Source: CAD feature listing. Evaluate the final solid. Frame: model axes, mm. A direction names the side the tool comes from. Give positions to 0.01 mm unless a question says otherwise; leave off trailing zeros. Loops run counter-clockwise (first coordinate to the right, second up) from the corner with the lowest first, then second, coordinate; pieces in that order, holes last. Notation, with made-up numbers: M 1.5,40.5 L 42.5,40.5 A3 ccw 42.5,45.5 Z; hole C 78.25,43 d10. An arc over 180 degrees is marked long. Put each result on its own line as item: value.
from build123d import *

# Parameters (mm, degrees)
F0_W     = 82
F0_H     = 60.5
F1_DEPTH = 2
F2_R     = 2.375
F3_DEPTH = 2
F4_DEPTH = 4
F5_DEPTH = 2
F6_W     = 2
F6_H     = 10.75
F7_DEPTH = 10.501
F8_W     = 0.5
F8_H     = 10
F9_DEPTH = 5


with BuildPart() as f1:
    # F0 (on Top) → F1 (new body)
    with BuildSketch(Plane.XY):
        Rectangle(F0_W, F0_H)
    extrude(amount=F1_DEPTH)

    # F2 (on face) → F3 (join)
    with BuildSketch(Plane.YZ.offset(41)):
        Polygon((19.5, 2), (-19.5, 2), (-30.25, 2), (-30.25, 0), (30.25, 0), (30.25, 2), align=None)
        with BuildLine():
            Line((19.5, 7.125), (19.5, 2))
            Line((19.5, 2), (30.25, 2))
            Line((30.25, 2), (30.25, 7.125))
            ThreePointArc((30.25, 7.125), (24.875, 12.5), (19.5, 7.125))
        make_face()
        with Locations((24.875, 7.125)):
            Circle(F2_R, mode=Mode.SUBTRACT)
    extrude(amount=F3_DEPTH)

    # F2 (on face) → F4 (join)
    with BuildSketch(Plane.YZ.offset(41)):
        with BuildLine():
            Line((-30.25, 2), (-19.5, 2))
            Line((-19.5, 2), (-19.5, 7.125))
            ThreePointArc((-19.5, 7.125), (-24.875, 12.5), (-30.25, 7.125))
            Line((-30.25, 7.125), (-30.25, 2))
        make_face()
        with Locations((-24.875, 7.125)):
            Circle(F2_R, mode=Mode.SUBTRACT)
    extrude(amount=F4_DEPTH)

    # F5 (add): a face of the model
    f5_faces = [f1.faces().sort_by_distance(p)[0] for p in [
        (44, -24.875, 2),
    ]]
    extrude(f5_faces, amount=F5_DEPTH)

    # F6 (on face) → F7 (cut, through all)
    with BuildSketch(Plane.XY.offset(2)):
        with Locations((42, -24.875)):
            Rectangle(F6_W, F6_H)
    extrude(amount=F7_DEPTH, mode=Mode.SUBTRACT)

    # F8 (on face) → F9 (cut)
    with BuildSketch(Plane.YZ.offset(45)):
        with Locations((-30, 5)):
            Rectangle(F8_W, F8_H)
    extrude(amount=-F9_DEPTH, mode=Mode.SUBTRACT)


solid = f1.part
1. Section query D-D (x = -22.5). Output: boundary loops of the cut face in (y, z).
Found:
outline: M -30.25,0 L 30.25,0 L 30.25,2 L -30.25,2 Z
2. Contact query for flat-ended pins moving along their axis: P1, Ø0.6, axis at x = 44.5, z = 3, coming from the +Y side; P2, Ø4.5, axis at y = 24.875, z = 7.125, coming from the +X side; P3, Ø3, axis at y = 18.5, z = 3.5, coming from the +X side; P4, Ø1, axis at x = -5, y = -19, coming from the +Z side. Output: stop coordinate, or through.
Found:
P1: y = -19.5
P2: through
P3: x = 43
P4: z = 2
3. Material intervals for line 1 (Z direction, x = -34, y = 27.5); line 2 (X direction, y = 21.5, z = 9.5), sorted ascending. Write a range as from..to.
Found:
line 1: 0..2
line 2: 41..43
4. Section query A-A (z = 6.25). Output: boundary loops of the cut face in (x, y).
Found:
outline: M 41,19.5 L 43,19.5 L 43,22.67 L 41,22.67 Z; M 41,27.08 L 43,27.08 L 43,30.25 L 41,30.25 Z; M 43,-29.75 L 45,-29.75 L 45,-27.08 L 43,-27.08 Z; M 43,-22.67 L 45,-22.67 L 45,-19.5 L 43,-19.5 Z
5. Section query C-C (y = 21). Output: boundary loops of the cut face in (x, z), plus the area to 3 significant figures.
Found:
outline: M -41,0 L 43,0 L 43,10.85 L 41,10.85 L 41,2 L -41,2 Z
area: 186 mm^2
6. Access query for faces 4 (the flat face through (43, 14.5, 1.6)), 5 (the flat face through (42, 19.5, 5)), 6 (the flat face through (44, -29.75, 4)), 7 (the flat face through (43, -23.6, 4.8)). Directions: +Z, -Z, +X, -X, +Y, -Y. A direction counts if a zero-diameter tool reaches every point of the face in a straight line with its end or side. Return the directions, or none.
Found:
face 4: +Z, -Z, +X, +Y
face 5: +Z, +X, -X, -Y
face 6: +Z, -Z, +X, -Y
face 7: +Z, -X, -Y
7. Section query B-B (z = 10.75). Output: boundary loops of the cut face in (x, y).
Found:
outline: M 41,20.91 L 43,20.91 L 43,28.84 L 41,28.84 Z; M 43,-28.84 L 45,-28.84 L 45,-20.91 L 43,-20.91 Z
8. Draft query along Z for faces 1 (the cylindrical face through (43.99, -26.76, 5.68)), 2 (the flat face through (1, 0, 0)), 3 (the flat face through (41, 22, 7)). Return one class per face: pulls with the +Z half, pulls with the -Z half, needs draft (parallel to the pull), parting line crosses it, or undercut.
Found:
face 1: undercut
face 2: pulls with the -Z half
face 3: needs draft
